CAD build for the part. Positions are in the model's coordinates, mm. A direction names the side the tool comes from. Round coordinates to 2 decimals unless told otherwise and drop trailing zeros. Order: outer loops, then holes, each group sorted by start corner. A loop starts at its lowest first (then second) coordinate and runs counter-clockwise, first axis right, second up. Notation, with made-up numbers: M 32.25,27 L 70.25,27 A17 cw 70.25,41 Z; hole C -15,-14 d11. An arc over 180 degrees is marked long. Answer as a JSON object with one key per item and string values.
```python
from build123d import *

# Parameters (mm, degrees)
F2_R            = 1.25
F3_DEPTH        = 5
F3_COPIES_COUNT = 3
F5_D            = 2.6
F5_CBORE_D      = 5
F5_CBORE_DEPTH  = 4
F5_COPIES_COUNT = 3
F6_W            = 3
F6_H            = 3


# Not quite as in the source:
# - a pattern or mirror of a feature is missing from the dataset's text; its kind, count and spacing are read off the source's solid


with BuildPart() as f1:
    # F0 (on Front) → F1 (revolve)
    with BuildSketch(Plane.XZ):
        Polygon((10, 4), (10, 0), (30, 0), (30, 8), (15, 8), (15, 4), align=None)
    revolve(axis=Axis((0, 0, 1.9594207406), (0, 0, -1)))

    # F2 (on face) → F3 (join)
    with BuildSketch(Plane.XY.offset(8)):
        with Locations((20, 0)):
            Circle(F2_R)
    f3 = extrude(amount=F3_DEPTH)

    # F3_copies: F3 ×3 about axis
    f3_copies_axis = Axis((0, 0, 0), (0, 0, 1))
    for i in range(1, F3_COPIES_COUNT):
        add(f3.rotate(f3_copies_axis, i * 360 / F3_COPIES_COUNT))

    # F5 (through all)
    with Locations(Plane(origin=(0, 0, 0), x_dir=(1, 0, 0), z_dir=(0, 0, -1))):
        with Locations((-20, 0)):
            f5 = CounterBoreHole(F5_D / 2, F5_CBORE_D / 2, F5_CBORE_DEPTH)

    # F5_copies: F5 ×3 about axis
    f5_copies_axis = Axis((0, 0, 0), (0, 0, 1))
    for i in range(1, F5_COPIES_COUNT):
        add(f5.rotate(f5_copies_axis, i * 360 / F5_COPIES_COUNT), mode=Mode.SUBTRACT)

    # F6 (on Front) → F7 (revolve, cut)
    with BuildSketch(Plane.XZ):
        with Locations((28.5, 6.5)):
            Rectangle(F6_W, F6_H)
    revolve(axis=Axis((0, 0, 1.9594207406), (0, 0, -1)), mode=Mode.SUBTRACT)


solid = f1.part
```
Item 1: Drop flat-ended pins along their axis: pin 1 Ø10 at (x, y) = (-3.5, 4) entering from -Z; pin 2 Ø3 at (x, y) = (10, 17.32) entering from -Z; pin 3 Ø4.5 at (x, y) = (10, 17.32) entering from +Z; pin 4 Ø6 at (y, z) = (19, 4.5) entering from +X. Give the stop position or say it passes through.
Worked answers:
{"pin 1": "stops at z = 0", "pin 2": "stops at z = 4", "pin 3": "stops at z = 8", "pin 4": "stops at x = 25.38"}
Item 2: Wall check: line 1 along Y through (x, z) = (0, 5.5); line 2 along Z through (x, y) = (-9, 26); line 3 along Z through (x, y) = (14, 0.5). Give the ranges that are in metal, low to high. Write a range as [from, to].
Worked answers:
{"line 1": "y = [-27, -15], [15, 27]", "line 2": "z = [0, 5]", "line 3": "z = [0, 4]"}
Item 3: Saw through at D-D on y = 23.5. List the corners of the cut face in (x, z), and give its area (3 significant figures).
Worked answers:
{"outline": "M -18.65,0 L 18.65,0 L 18.65,5 L 13.29,5 L 13.29,8 L -13.29,8 L -13.29,5 L -18.65,5 Z", "area": "266 mm2"}
Item 4: Saw through at B-B on x = -20. List the corners of the cut face in (y, z), and give its area (3 significant figures).
Worked answers:
{"outline": "M -22.36,0 L -2.5,0 L -2.5,4 L -1.3,4 L -1.3,8 L -18.14,8 L -18.14,5 L -22.36,5 Z; M 1.3,4 L 2.5,4 L 2.5,0 L 22.36,0 L 22.36,5 L 18.14,5 L 18.14,8 L 1.3,8 Z", "area": "302 mm2"}
Item 5: Saw through at C-C on y = 8.5. List the corners of the cut face in (x, z), and give its area (3 significant figures).
Worked answers:
{"outline": "M -28.77,0 L -5.27,0 L -5.27,4 L -12.36,4 L -12.36,8 L -25.63,8 L -25.63,5 L -28.77,5 Z; M 5.27,0 L 28.77,0 L 28.77,5 L 25.63,5 L 25.63,8 L 12.36,8 L 12.36,4 L 5.27,4 Z", "area": "300 mm2"}
Item 6: Two-plate mould, pull along Y, no slides. Class faces 4 (the cylindrical face through (-10.16, 18.56, 10.46)), 5 (the cylindrical face through (-29.97, -1.32, 2.54)), 6 (the cylindrical face through (9.4, 18.474, 6.028)), 7 (the flat face through (-10, 17, 13)): released by +Y, released by -Y, zero draft, split by the parting line, or undercut.
Worked answers:
{"face 4": "undercut", "face 5": "split by the parting line", "face 6": "undercut", "face 7": "zero draft"}
Item 7: 3-axis set-ups, long thin cutter, end or side, ignore diameter. For faces 1 (the flat face through (25, -11, 5)), 2 (the flat face through (8.5, -16.9, 4)), 3 (the cylindrical face through (-18.7, -0.06, 6.03)): which of +Z, -Z, +X, -X, +Y, -Y reach the whole face in a straight line?
Worked answers:
{"face 1": "+Z", "face 2": "-Z", "face 3": "+Z, -Z"}
Item 8: Saw through at A-A on y = 0. List the corners of the cut face in (x, z).
Worked answers:
{"outline": "M -30,0 L -22.5,0 L -22.5,4 L -21.3,4 L -21.3,8 L -27,8 L -27,5 L -30,5 Z; M -18.7,4 L -17.5,4 L -17.5,0 L -10,0 L -10,4 L -15,4 L -15,8 L -18.7,8 Z; M 10,0 L 30,0 L 30,5 L 27,5 L 27,8 L 21.25,8 L 21.25,13 L 18.75,13 L 18.75,8 L 15,8 L 15,4 L 10,4 Z"}
